Source: CAD feature listing. Evaluate the final solid. Frame: model axes, mm. Face numbers are marked on the shaded views. A direction names the side the tool comes from. Round coordinates to 2 decimals unless told otherwise and drop trailing zeros. Loops run counter-clockwise (first coordinate to the right, second up) from the corner with the lowest first, then second, coordinate; pieces in that order, holes last. Notation, with made-up numbers: M 80.25,-15 L 90.25,-15 A30 cw 90.25,13 Z; hole C 1,-14 d11. An arc over 180 degrees is marked long. Write each question's results on one line, items separated by ' | '. Start each with the question number.
1. Ray query, line 1 (Y direction, x = 0, z = 13); line 2 (X direction, y = -44, z = -45.5); line 3 (Y direction, x = 51, z = -73.5). Return the intervals inside material, ascending.
2. Section A-A on y = -9. Output: boundary loops of the cut face in (x, z).
3. Set-up query: the marked faces 1 and 2. Return all of +Z, -Z, +X, -X, +Y, -Y with unobstructed straight access to the full face (end or side cutting, diameter ignored); none if empty.
4. Section C-C on z = 31.5. Output: boundary loops of the cut face in (x, y), and give its area (3 significant figures).
5. Section B-B on x = 0. Output: boundary loops of the cut face in (y, z), and give its area (3 significant figures).
from build123d import *

# Parameters (mm, degrees)
BOSS_EXTRUDE1_DEPTH     = 105
SKETCH2_R               = 11
CUT_EXTRUDE1_DEPTH      = 106
CUT_EXTRUDE1_DEPTH_BACK = 106


with BuildPart() as part:
    # Sketch1 → Boss-Extrude1 (new body, symmetric)
    with BuildSketch(Plane.XY):
        Polygon((350, 232.421392473), (-350, 232.421392473), (-350, -67.578607527), (-65, -67.578607527), (-55, -57.578607527), (-55, 81.421392473), (55, 81.421392473), (55, -57.578607527), (65, -67.578607527), (350, -67.578607527), align=None)
    extrude(amount=BOSS_EXTRUDE1_DEPTH, both=True)

    # Sketch2 → Cut-Extrude1 (cut, two sides)
    with BuildSketch(Plane.XY) as cut_extrude1_sk:
        with Locations((0, 172.421392473)):
            Circle(SKETCH2_R)
    extrude(amount=CUT_EXTRUDE1_DEPTH, mode=Mode.SUBTRACT)
    extrude(cut_extrude1_sk.sketch, amount=-CUT_EXTRUDE1_DEPTH_BACK, mode=Mode.SUBTRACT)


solid = part.part
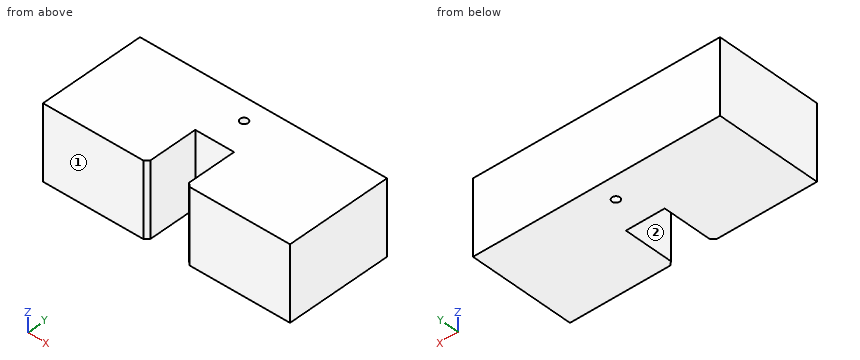
Taken from the geometry:
1) line 1: 81.42 to 161.42, 183.42 to 232.42 | line 2: -350 to -55, 55 to 350 | line 3: 81.42 to 232.42
2) outline: M -350,-105 L -55,-105 L -55,105 L -350,105 Z; M 55,-105 L 350,-105 L 350,105 L 55,105 Z
3) face 1: +Z, -Z, +X, -X, -Y | face 2: +Z, -Z, -Y
4) outline: M -350,-67.58 L -65,-67.58 L -55,-57.58 L -55,81.42 L 55,81.42 L 55,-57.58 L 65,-67.58 L 350,-67.58 L 350,232.42 L -350,232.42 Z; hole C 0,172.42 d22 | area: 193,000 mm^2
5) outline: M 81.42,-105 L 161.42,-105 L 161.42,105 L 81.42,105 Z; M 183.42,-105 L 232.42,-105 L 232.42,105 L 183.42,105 Z | area: 27,100 mm^2
